CAD build for the part. Positions are in the model's coordinates, mm. Face numbers are marked on the shaded views. A direction names the side the tool comes from. Give positions to 0.01 mm unless a question says otherwise; leave off trailing zeros. Loops run counter-clockwise (first coordinate to the right, second up) from the corner with the lowest first, then second, coordinate; pieces in that order, holes last. Notation, with made-up numbers: M -19.75,-4 L 39.25,-4 A22 cw 39.25,2 Z; hole C 61.25,53.5 d4. An arc over 180 degrees is marked long. Answer as CSV lines item,"result".
```python
from build123d import *

# Parameters (mm, degrees)
SKETCH1_W           = 70
SKETCH1_H           = 100
BOSS_EXTRUDE1_DEPTH = 5
SKETCH2_W           = 13
SKETCH2_H           = 20
BOSS_EXTRUDE2_DEPTH = 5
SKETCH4_W           = 8.5
SKETCH4_H           = 23.6
BOSS_EXTRUDE3_DEPTH = 19
SKETCH5_R           = 1.5
CUT_EXTRUDE1_DEPTH  = 26
SKETCH6_W           = 13
SKETCH6_H           = 20
BOSS_EXTRUDE4_DEPTH = 8.385
SKETCH7_R           = 8
CUT_EXTRUDE2_DEPTH  = 63
CUT_EXTRUDE3_REACH  = 7
SKETCH8_R           = 2.5


with BuildPart() as part:
    # Sketch1 → Boss-Extrude1 (new body)
    with BuildSketch(Plane(origin=(0, 0, 0), x_dir=(1, 0, 0), z_dir=(0, 1, 0))):
        Rectangle(SKETCH1_W, SKETCH1_H)
    extrude(amount=BOSS_EXTRUDE1_DEPTH)

    # Sketch2 → Boss-Extrude2 (add)
    with BuildSketch(Plane(origin=(0, 5, 0), x_dir=(1, 0, 0), z_dir=(0, 1, 0))):
        Polygon((-15.28967138, -11.9), (-25.28967138, -11.9), (-25.28967138, -35.5), (25.5, -35.5), (25.5, -11.9), (15.5, -11.9), (15.5, -4.5), (-15.28967138, -4.5), align=None)
        with Locations((-23, 31)):
            Rectangle(SKETCH2_W, SKETCH2_H)
        with Locations((9, 31)):
            Rectangle(SKETCH2_W, SKETCH2_H)
    extrude(amount=BOSS_EXTRUDE2_DEPTH)

    # Sketch4 → Boss-Extrude3 (add)
    with BuildSketch(Plane(origin=(0, 10, 0), x_dir=(1, 0, 0), z_dir=(0, 1, 0))):
        with Locations((-21.03967138, -23.7)):
            Rectangle(SKETCH4_W, SKETCH4_H)
        with Locations((21.25, -23.7)):
            Rectangle(SKETCH4_W, SKETCH4_H)
    extrude(amount=BOSS_EXTRUDE3_DEPTH)

    # Sketch5 → Cut-Extrude1 (cut)
    with BuildSketch(Plane(origin=(0, 0, 11.9), x_dir=(-1, 0, 0), z_dir=(0, 0, -1))):
        with Locations((19.39, 22.5)):
            Circle(SKETCH5_R)
        with Locations((19.39, 14.63)):
            Circle(SKETCH5_R)
        with Locations((-19.5, 22.5)):
            Circle(SKETCH5_R)
        with Locations((-19.5, 14.63)):
            Circle(SKETCH5_R)
    extrude(amount=-CUT_EXTRUDE1_DEPTH, mode=Mode.SUBTRACT)

    # Sketch6 → Boss-Extrude4 (add)
    with BuildSketch(Plane(origin=(0, 10, 0), x_dir=(1, 0, 0), z_dir=(0, 1, 0))):
        with Locations((-23, 31)):
            Rectangle(SKETCH6_W, SKETCH6_H)
        with Locations((9, 31)):
            Rectangle(SKETCH6_W, SKETCH6_H)
    extrude(amount=BOSS_EXTRUDE4_DEPTH)

    # Sketch7 → Cut-Extrude2 (cut)
    with BuildSketch(Plane.ZY.offset(29.5)):
        with Locations((-31, 18)):
            Circle(SKETCH7_R)
    extrude(amount=-CUT_EXTRUDE2_DEPTH, mode=Mode.SUBTRACT)

    # Sketch8 → Cut-Extrude3 (cut, up to next)
    with BuildSketch(Plane(origin=(0, 5, 0), x_dir=(1, 0, 0), z_dir=(0, 1, 0)), mode=Mode.PRIVATE) as cut_extrude3_sk1:
        with Locations((30, 45)):
            Circle(SKETCH8_R)
    cut_extrude3_tool1 = extrude(cut_extrude3_sk1.sketch, amount=-CUT_EXTRUDE3_REACH, mode=Mode.PRIVATE) & part.part
    add(cut_extrude3_tool1.solids().sort_by_distance((30, 5, -45))[0], mode=Mode.SUBTRACT)
    # Sketch8 → Cut-Extrude3 (cut, up to next)
    with BuildSketch(Plane(origin=(0, 5, 0), x_dir=(1, 0, 0), z_dir=(0, 1, 0)), mode=Mode.PRIVATE) as cut_extrude3_sk2:
        with Locations((-30, 45)):
            Circle(SKETCH8_R)
    cut_extrude3_tool2 = extrude(cut_extrude3_sk2.sketch, amount=-CUT_EXTRUDE3_REACH, mode=Mode.PRIVATE) & part.part
    add(cut_extrude3_tool2.solids().sort_by_distance((-30, 5, -45))[0], mode=Mode.SUBTRACT)
    # Sketch8 → Cut-Extrude3 (cut, up to next)
    with BuildSketch(Plane(origin=(0, 5, 0), x_dir=(1, 0, 0), z_dir=(0, 1, 0)), mode=Mode.PRIVATE) as cut_extrude3_sk3:
        with Locations((-30, -45)):
            Circle(SKETCH8_R)
    cut_extrude3_tool3 = extrude(cut_extrude3_sk3.sketch, amount=-CUT_EXTRUDE3_REACH, mode=Mode.PRIVATE) & part.part
    add(cut_extrude3_tool3.solids().sort_by_distance((-30, 5, 45))[0], mode=Mode.SUBTRACT)
    # Sketch8 → Cut-Extrude3 (cut, up to next)
    with BuildSketch(Plane(origin=(0, 5, 0), x_dir=(1, 0, 0), z_dir=(0, 1, 0)), mode=Mode.PRIVATE) as cut_extrude3_sk4:
        with Locations((30, -45)):
            Circle(SKETCH8_R)
    cut_extrude3_tool4 = extrude(cut_extrude3_sk4.sketch, amount=-CUT_EXTRUDE3_REACH, mode=Mode.PRIVATE) & part.part
    add(cut_extrude3_tool4.solids().sort_by_distance((30, 5, 45))[0], mode=Mode.SUBTRACT)


solid = part.part
```
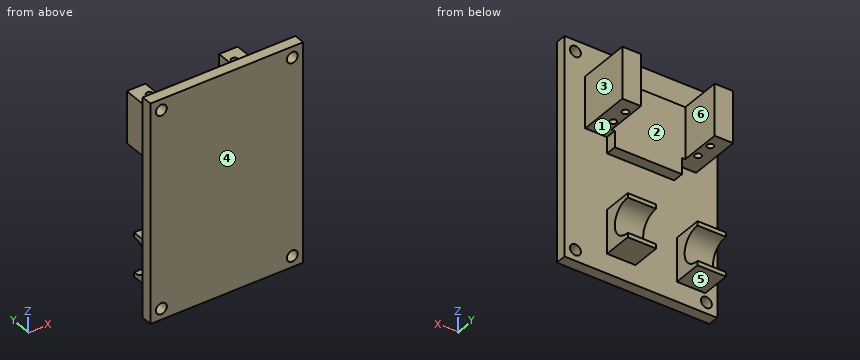
Q1. Cut at D-D (x = 5). Write the cut outline in (y, z) (3 decimals), and give its area (3 significant figures).
Solution:
outline,"M 0,-50 L 5,-50 L 5,-41 L 18.385,-41 L 18.385,-38.991 A8 cw long 18.385,-23.009 L 18.385,-21 L 5,-21 L 5,4.5 L 10,4.5 L 10,35.5 L 5,35.5 L 5,50 L 0,50 Z"
area,"816 mm²"
Q2. Wall check: line 1 (Y direction, x = -19.39, z = 29.75); line 2 (X direction, y = 3.3, z = -45); line 3 (Y direction, x = -19, z = 23). Give the ranges that are in metal, low to high. Write a range as [from, to].
Solution:
line 1,"y = [0, 13.13], [16.13, 21], [24, 29]"
line 2,"x = [-35, -32.5], [-27.5, 27.5], [32.5, 35]"
line 3,"y = [0, 13.18], [16.08, 21.05], [23.95, 29]"
Q3. Pin check, flat tips, straight feed: P1, Ø8, axis at x = -22, y = 19, coming from the -Z side; P2, Ø12, axis at x = 11, z = -8, coming from the +Y side; P3, Ø3, axis at x = 30, z = -45, coming from the +Y side; P4, Ø1.5, axis at x = -2, y = 7, coming from the -Z side. Stop position of each tip, or through.
Solution:
P1,"stops at z = -41"
P2,"stops at y = 5"
P3,"passes through"
P4,"stops at z = 4.5"
Q4. Mould opens along X. For the marked faces 1, 2 and 3 say: released by +X, released by -X, zero draft, split by the parting line, or undercut.
Solution:
face 1,"zero draft"
face 2,"undercut"
face 3,"released by +X"
Q5. Cut at A-A (y = 22.5). Write the cut outline in (x, z), and give its area (3 significant figures).
Solution:
outline,"M -25.29,11.9 L -20.89,11.9 L -20.89,35.5 L -25.29,35.5 Z; M -17.89,11.9 L -16.79,11.9 L -16.79,35.5 L -17.89,35.5 Z; M 17,11.9 L 18,11.9 L 18,35.5 L 17,35.5 Z; M 21,11.9 L 25.5,11.9 L 25.5,35.5 L 21,35.5 Z"
area,"260 mm²"
Q6. Cut at B-B (z = 13.5). Write the cut outline in (x, y), and give its area (3 significant figures).
Solution:
outline,"M -35,0 L 35,0 L 35,5 L 25.5,5 L 25.5,29 L 17,29 L 17,10 L -16.79,10 L -16.79,29 L -25.29,29 L -25.29,5 L -35,5 Z; hole C -19.39,14.63 d3; hole C -19.39,22.5 d3; hole C 19.5,14.63 d3; hole C 19.5,22.5 d3"
area,"899 mm²"
Q7. Cut at C-C (z = -31). Write the cut outline in (x, y).
Solution:
outline,"M -35,0 L 35,0 L 35,5 L 15.5,5 L 15.5,10 L 2.5,10 L 2.5,5 L -16.5,5 L -16.5,10 L -29.5,10 L -29.5,5 L -35,5 Z"
Q8. Which spindle directions (+Z, -Z, +X, -X, +Y, -Y) get a long thin tool onto all of the face, cutting with end or side? Do the marked faces 4, 5 and 6. Say none if no direction does.
Solution:
face 4,"+Z, -Z, +X, -X, -Y"
face 5,"-Z, +X, -X, +Y"
face 6,"+Z, +Y"
